Can you work these out from the model? Positions are in its coordinate system, mm. Face numbers are marked on the shaded views. A direction names the side the tool comes from. Round coordinates to 2 decimals unless told otherwise and drop trailing zeros. Loops run counter-clockwise (first coordinate to the right, second up) from the corner with the lowest first, then second, coordinate; pieces in that order, holes last. Notation, with made-up numbers: (37, 8.5) -> (67, 8.5) arc R7 cw to (67, 12.5) -> close; hole circle Ø8 at (20.25, 16.25). An arc over 180 degrees is marked (long way). Use a Markdown table: item, result.
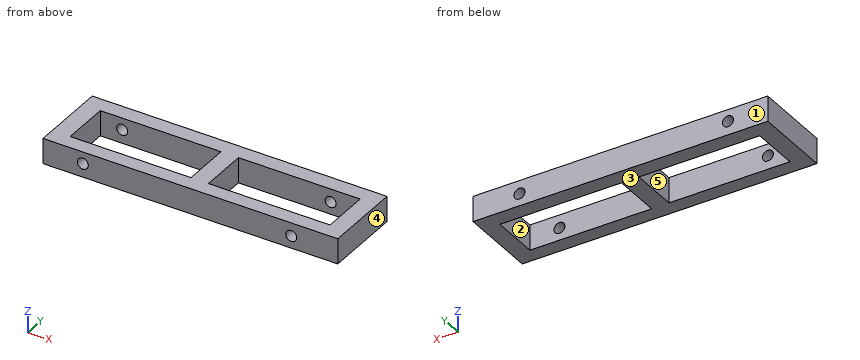
from build123d import *

# Parameters (mm, degrees)
F0_W     = 150.861204
F0_H     = 40.061776
F1_DEPTH = 13
F2_W     = 133.00509
F2_H     = 24.494914
F3_DEPTH = 25
F4_W     = 8.928052
F4_H     = 32.736194
F5_DEPTH = 13
F7_D     = 5.6


with BuildPart() as f1:
    # F0 (on Top) → F1 (new body)
    with BuildSketch(Plane.XY):
        Rectangle(F0_W, F0_H)
    extrude(amount=F1_DEPTH)

    # F2 (on face) → F3 (cut)
    with BuildSketch(Plane.XY.offset(13)):
        with Locations((0.228923, -0.228925)):
            Rectangle(F2_W, F2_H)
    extrude(amount=-F3_DEPTH, mode=Mode.SUBTRACT)

    # F4 (on face) → F5 (join)
    with BuildSketch(Plane.XY.offset(13)):
        Rectangle(F4_W, F4_H)
    extrude(amount=-F5_DEPTH)

    # F7 (through all)
    with Locations(Plane(origin=(0, 20.030888, 0), x_dir=(-1, 0, 0), z_dir=(0, 1, 0))):
        with Locations((55.056326, 6.982195), (-51.622458, 6.295422)):
            Hole(F7_D / 2)


solid = f1.part
1. Will these pins go through, and if not, where does the flat tip stop? pin 1 Ø5 at (x, z) = (-55.06, 6.98) entering from +Y; pin 2 Ø10 at (x, y) = (-36.5, -14.5) entering from -Z.
Answer sheet:
| item | result |
|---|---|
| pin 1 | passes through |
| pin 2 | stops at z = 0 |
2. I need wall thicknesses on line 1 (X direction, y = -12, z = 7.5); line 2 (Y direction, x = -31, z = 6.5); line 3 (X direction, y = 18.5, z = 7.5). Which ranges of each line are inside material? Lowest first, please.
Answer sheet:
| item | result |
|---|---|
| line 1 | x = -75.43 to -66.27, -4.46 to 4.46, 66.73 to 75.43 |
| line 2 | y = -20.03 to -12.48, 12.02 to 20.03 |
| line 3 | x = -75.43 to -57.81, -52.3 to 49.09, 54.15 to 75.43 |
3. I want a section at C-C (z = 2). Please give me the cut outline in (x, y).
Answer sheet:
| item | result |
|---|---|
| outline | (-75.43, -20.03) -> (75.43, -20.03) -> (75.43, 20.03) -> (-75.43, 20.03) -> close; hole (-66.27, -12.48) -> (-4.46, -12.48) -> (-4.46, 12.02) -> (-66.27, 12.02) -> close; hole (4.46, -12.48) -> (66.73, -12.48) -> (66.73, 12.02) -> (4.46, 12.02) -> close |
4. If we mould it in two halves opening along Y, with no side actions, what happens to the marked faces 1, 2 and 3? For each: +Y half, -Y half, draft (parallel to the pull), parting line (faces both ways), or undercut.
Answer sheet:
| item | result |
|---|---|
| face 1 | +Y half |
| face 2 | undercut |
| face 3 | draft |
5. I want a section at D-D (x = -54.5). Please give me the cut outline in (y, z).
Answer sheet:
| item | result |
|---|---|
| outline | (-20.03, 0) -> (-12.48, 0) -> (-12.48, 4.24) -> (-20.03, 4.24) -> close; (-20.03, 9.73) -> (-12.48, 9.73) -> (-12.48, 13) -> (-20.03, 13) -> close; (12.02, 0) -> (20.03, 0) -> (20.03, 4.24) -> (12.02, 4.24) -> close; (12.02, 9.73) -> (20.03, 9.73) -> (20.03, 13) -> (12.02, 13) -> close |
6. Which directions (+Z, -Z, +X, -X, +Y, -Y) give clear straight access to the entire face, cutting with the end or side of a thin tool? Please do the marked faces 4 and 5.
Answer sheet:
| item | result |
|---|---|
| face 4 | +Z, -Z, +X, +Y, -Y |
| face 5 | +Z, -Z |
7. I want a section at B-B (y = -5). Please give me the cut outline in (x, z).
Answer sheet:
| item | result |
|---|---|
| outline | (-75.43, 0) -> (-66.27, 0) -> (-66.27, 13) -> (-75.43, 13) -> close; (-4.46, 0) -> (4.46, 0) -> (4.46, 13) -> (-4.46, 13) -> close; (66.73, 0) -> (75.43, 0) -> (75.43, 13) -> (66.73, 13) -> close |
8. I want a section at A-A (x = 38.5). Please give me the cut outline in (y, z), plus the area to 3 significant figures.
Answer sheet:
| item | result |
|---|---|
| outline | (-20.03, 0) -> (-12.48, 0) -> (-12.48, 13) -> (-20.03, 13) -> close; (12.02, 0) -> (20.03, 0) -> (20.03, 13) -> (12.02, 13) -> close |
| area | 202 mm² |
